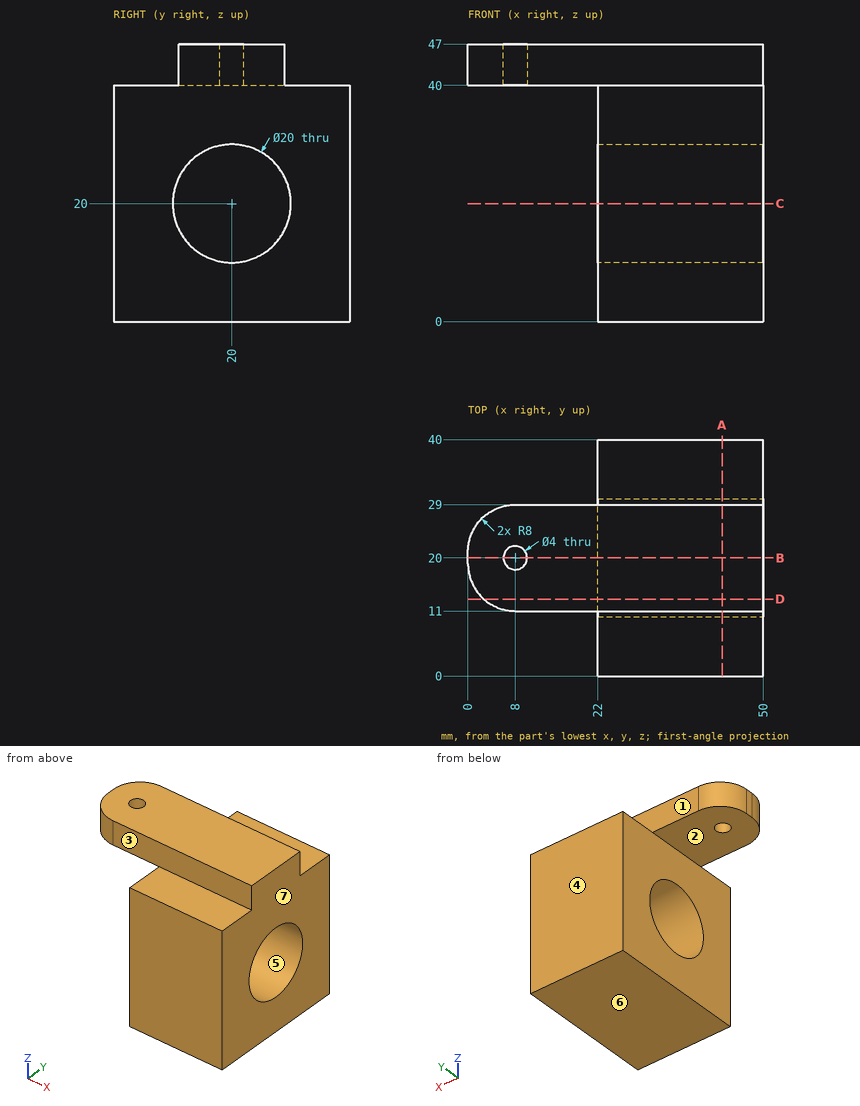
Drawing for the job (mm, zero at the part's lowest x, y, z). A direction names the side the tool comes from. Round coordinates to 2 decimals unless told otherwise and drop trailing zeros. Order: outer loops, then holes, each group sorted by start corner. A loop starts at its lowest first (then second) coordinate and runs counter-clockwise, first axis right, second up. Notation, with made-up numbers: (79.5, -8.75) -> (99.5, -8.75) arc R5 ccw to (99.5, -1.75) -> close; hole circle Ø3 at (27, 31.5). An arc over 180 degrees is marked (long way). Write item = value, one per line. Start each with the question number.
(1) Pin check, flat tips, straight feed: P1, Ø6, axis at y = 11, z = 18.5, coming from the -X side; P2, Ø12, axis at x = 41.5, y = 3.5, coming from the +Z side; P3, Ø5.5, axis at x = 19.5, z = 44, coming from the -Y side. Stop position of each tip, or through.
(2) Cut at C-C, the plane z = 20. List the corners of the cut face in (x, y), then the cut area to 3 significant figures.
(3) Cut at A-A, the plane x = 43. List the corners of the cut face in (y, z).
(4) Cut at B-B, the plane y = 20. List the corners of the cut face in (x, z).
(5) Which spindle directions (+Z, -Z, +X, -X, +Y, -Y) get a long thin tool onto all of the face, cutting with end or side? Do the marked faces 1, 2, 3 and 4. Say none if no direction does.
(6) Cut at D-D, the plane y = 13. List the corners of the cut face in (x, z), then the cut area to 3 significant figures.
(7) Pull direction Z, two halves, no side cores. Call the marked faces 5, 6 and 7: released by +Z, released by -Z, zero draft, split by the parting line, or undercut.
(8) Probe line 1 (Y direction, x = 8, z = 42); line 2 (Y direction, x = 28, z = 20); line 3 (Z direction, x = 47.5, y = 32). List the from-to ranges inside material, lowest first. Write a range as [from, to].
Model answer:
q1.P1 = 22
q1.P2 = 40
q1.P3 = 11
q2.outline = (22, 0) -> (50, 0) -> (50, 10) -> (22, 10) -> close; (22, 30) -> (50, 30) -> (50, 40) -> (22, 40) -> close
q2.area = 560 mm2
q3.outline = (0, 0) -> (40, 0) -> (40, 40) -> (29, 40) -> (29, 47) -> (11, 47) -> (11, 40) -> (0, 40) -> close; hole circle Ø20 at (20, 20)
q4.outline = (0, 40) -> (6, 40) -> (6, 47) -> (0, 47) -> close; (10, 40) -> (22, 40) -> (22, 30) -> (50, 30) -> (50, 47) -> (10, 47) -> close; (22, 0) -> (50, 0) -> (50, 10) -> (22, 10) -> close
q5.face_1 = +Z, +X, -X, +Y
q5.face_2 = -Z, -X, +Y, -Y
q5.face_3 = +Z, +X, -X, -Y
q5.face_4 = +Z, -Z, +X, -X, +Y
q6.outline = (2.71, 40) -> (22, 40) -> (22, 27.14) -> (50, 27.14) -> (50, 47) -> (2.71, 47) -> close; (22, 0) -> (50, 0) -> (50, 12.86) -> (22, 12.86) -> close
q6.area = 1,050 mm2
q7.face_5 = undercut
q7.face_6 = released by -Z
q7.face_7 = zero draft
q8.line_1 = [11, 18], [22, 29]
q8.line_2 = [0, 10], [30, 40]
q8.line_3 = [0, 40]
